from build123d import *

# Parameters (mm, degrees)
SKETCH1_W           = 33
SKETCH1_H           = 86
BOSS_EXTRUDE1_DEPTH = 8
FILLET1_R           = 4
CHAMFER1_SIZE       = 1
SKETCH2_R           = 3.3
SKETCH2_R_2         = 2.25
CUT_EXTRUDE1_DEPTH  = 8
SKETCH3_R           = 5.5
CUT_EXTRUDE2_DEPTH  = 4.2
CHAMFER3_SIZE       = 3.2
SKETCH4_R           = 4
CUT_EXTRUDE3_DEPTH  = 4.4


with BuildPart() as part:
    # Sketch1 → Boss-Extrude1 (new body)
    with BuildSketch(Plane(origin=(0, 0, 0), x_dir=(1, 0, 0), z_dir=(0, 1, 0))):
        Rectangle(SKETCH1_W, SKETCH1_H)
    extrude(amount=BOSS_EXTRUDE1_DEPTH)

    # Fillet1
    fillet1_edges = [part.edges().sort_by_distance(p)[0] for p in [
        (16.5, 4, 43),
        (-16.5, 4, 43),
        (-16.5, 4, -43),
        (16.5, 4, -43),
    ]]
    fillet(fillet1_edges, radius=FILLET1_R)

    # Chamfer1
    chamfer1_edges = [part.edges().sort_by_distance(p)[0] for p in [
        (-16.5, 0, 0),
        (-16.5, 8, 0),
        (16.5, 0, 0),
        (0, 0, 43),
        (0, 0, -43),
        (15.328427125, 0, 41.828427125),
        (-15.328427125, 0, 41.828427125),
        (15.328427125, 0, -41.828427125),
        (-15.328427125, 0, -41.828427125),
        (0, 8, -43),
        (16.5, 8, 0),
        (0, 8, 43),
        (15.328427125, 8, 41.828427125),
        (-15.328427125, 8, 41.828427125),
        (15.328427125, 8, -41.828427125),
        (-15.328427125, 8, -41.828427125),
    ]]
    chamfer(chamfer1_edges, length=CHAMFER1_SIZE)

    # Sketch2 → Cut-Extrude1 (cut)
    with BuildSketch(Plane(origin=(0, 8, 0), x_dir=(1, 0, 0), z_dir=(0, 1, 0))):
        with Locations((0, 25.5)):
            Circle(SKETCH2_R)
        with Locations((0, -9.5)):
            Circle(SKETCH2_R)
        with Locations((11, -20.3)):
            Circle(SKETCH2_R_2)
        with Locations((-11, -35.3)):
            Circle(SKETCH2_R_2)
    extrude(amount=-CUT_EXTRUDE1_DEPTH, mode=Mode.SUBTRACT)

    # Sketch3 → Cut-Extrude2 (cut)
    with BuildSketch(Plane(origin=(0, 8, 0), x_dir=(1, 0, 0), z_dir=(0, 1, 0))):
        with Locations((0, -9.5)):
            Circle(SKETCH3_R)
    extrude(amount=-CUT_EXTRUDE2_DEPTH, mode=Mode.SUBTRACT)

    # Chamfer3
    chamfer3_edges = [part.edges().sort_by_distance(p)[0] for p in [
        (-3.3, 8, -25.5),
    ]]
    chamfer(chamfer3_edges, length=CHAMFER3_SIZE)

    # Sketch4 → Cut-Extrude3 (cut)
    with BuildSketch(Plane.XZ):
        with Locations((11, 20.3)):
            Circle(SKETCH4_R)
        with Locations((-11, 35.3)):
            Circle(SKETCH4_R)
    extrude(amount=-CUT_EXTRUDE3_DEPTH, mode=Mode.SUBTRACT)


solid = part.part
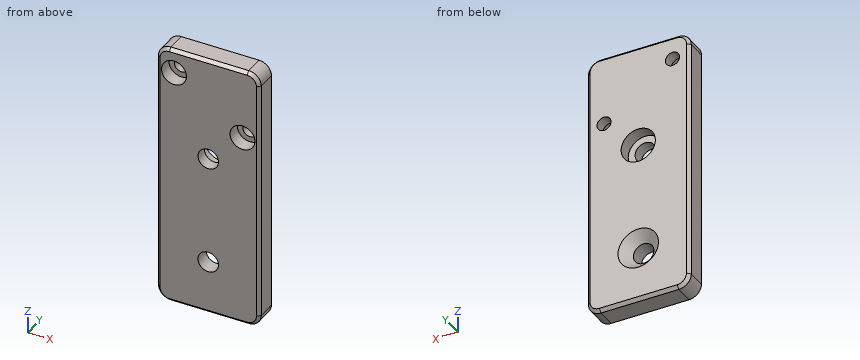
Part model, mm, in its own coordinate system. Round coordinates to 2 decimals unless told otherwise and drop trailing zeros. Loops run counter-clockwise (first coordinate to the right, second up) from the corner with the lowest first, then second, coordinate; pieces in that order, holes last. Notation, with made-up numbers: (-23, 0) - (-7, 0) arc R16 ccw to (-7, 17) - close; hole circle Ø4 at (42, 0.5). An arc over 180 degrees is marked (long way). Answer as a JSON object with one key per item and string values.
Item 1: Band-saw the part on B-B on x = -11. List the corners of the cut face in (y, z), plus the area to 3 significant figures.
Output:
{"outline": "(0, -42) - (1, -43) - (7, -43) - (8, -42) - (8, 33.05) - (4.4, 33.05) - (4.4, 31.3) - (0, 31.3) - close; (0, 39.3) - (4.4, 39.3) - (4.4, 37.55) - (8, 37.55) - (8, 42) - (7, 43) - (1, 43) - (0, 42) - close", "area": "635 mm2"}
Item 2: Band-saw the part on D-D on z = 9.5. List the corners of the cut face in (x, y).
Output:
{"outline": "(-16.5, 1) - (-15.5, 0) - (-3.3, 0) - (-3.3, 3.8) - (-5.5, 3.8) - (-5.5, 8) - (-15.5, 8) - (-16.5, 7) - close; (3.3, 0) - (15.5, 0) - (16.5, 1) - (16.5, 7) - (15.5, 8) - (5.5, 8) - (5.5, 3.8) - (3.3, 3.8) - close"}
Item 3: Band-saw the part on A-A on z = -25.5. List the corners of the cut face in (x, y), plus the area to 3 significant figures.
Output:
{"outline": "(-16.5, 1) - (-15.5, 0) - (-3.3, 0) - (-3.3, 4.8) - (-6.5, 8) - (-15.5, 8) - (-16.5, 7) - close; (3.3, 0) - (15.5, 0) - (16.5, 1) - (16.5, 7) - (15.5, 8) - (6.5, 8) - (3.3, 4.8) - close", "area": "199 mm2"}
Item 4: Band-saw the part on C-C on y = 6.25. List the corners of the cut face in (x, z).
Output:
{"outline": "(-16.5, -39) arc R4 ccw to (-12.5, -43) - (12.5, -43) arc R4 ccw to (16.5, -39) - (16.5, 39) arc R4 ccw to (12.5, 43) - (-12.5, 43) arc R4 ccw to (-16.5, 39) - close; hole circle Ø4.5 at (-11, 35.3); hole circle Ø11 at (0, 9.5); hole circle Ø9.5 at (0, -25.5); hole circle Ø4.5 at (11, 20.3)"}
Item 5: Pin check, flat tips, straight feed: pin 1 (4 mm diameter, centred on x = 11, z = 20.3, fed in from +Y); pin 2 (2.5 mm diameter, centred on x = -9.5, z = 36.5, fed in from -Y). Stop position of each tip, or through.
Output:
{"pin 1": "through", "pin 2": "y = 4.4"}
Item 6: Wall check: L1, parallel to Z at x = 0, y = 1; L2, parallel to X at y = 6.55, z = 20.3; L3, parallel to X at y = 3, z = 9.5. Give the ranges that are in metal, low to high.
Output:
{"L1": "-43 to -28.8, -22.2 to 6.2, 12.8 to 43", "L2": "-16.5 to 8.75, 13.25 to 16.5", "L3": "-16.5 to -3.3, 3.3 to 16.5"}
